Answer from the drawing. Dimensions are ordinates in mm from the lowest x, y and z of the part. A direction names the side the tool comes from. Round coordinates to 2 decimals unless told otherwise and drop trailing zeros. Loops run counter-clockwise (first coordinate to the right, second up) from the corner with the lowest first, then second, coordinate; pieces in that order, holes last.
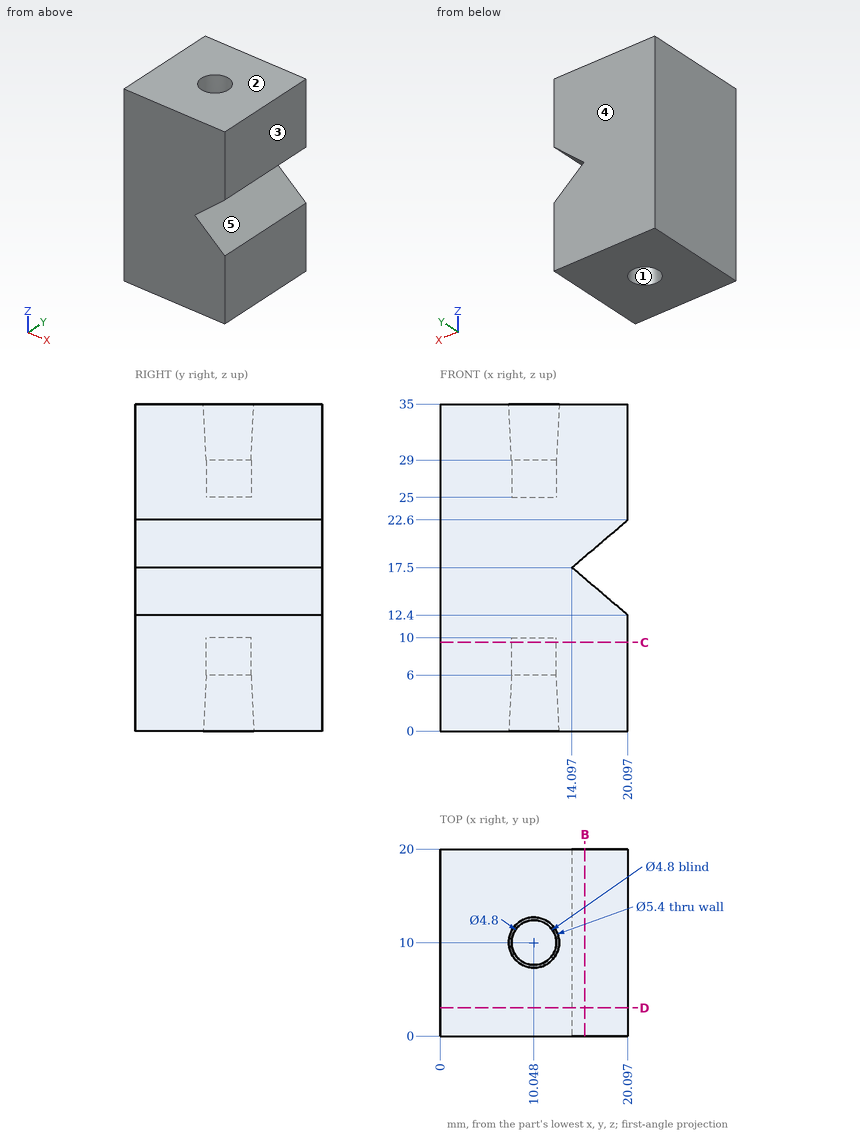
Item 1: For the marked faces 4 and 5, determine the directions among +Z, -Z, +X, -X, +Y, -Y from which every point of the face is accessible in a straight line to the end or side of a thin tool.
Item 2: Determine the mould class of the marked faces 1, 2 and 3 for opening direction X: pulls with the +X half, pulls with the -X half, needs draft (parallel to the pull), parting line crosses it, or undercut.
Item 3: Section B-B, the plane x = 15.5 is taken. Give the vertices of the cut face in (y, z).
Item 4: Section D-D, the plane y = 3 is taken. Give the vertices of the cut face in (x, z), plus the area to 3 significant figures.
Item 5: Straight lines are drawn through the part: line 1 (X direction, y = 11.25, z = 2.5) (1 decimal); line 2 (Y direction, x = 9.5, z = 8.5); line 3 (Z direction, x = 14.25, y = 4.75). For each, find the intervals that lie inside material, in ascending order.
Item 6: Each of these flat-tipped pins is pushed along its axis until it touches: P1, Ø3, axis at x = 10.05, y = 10, coming from the +Z side; P2, Ø2.5, axis at x = 10, y = 9, coming from the -Z side. Where does it stop, or does it pass through?
Item 7: Section C-C, the plane z = 9.5 is taken. Give the vertices of the cut face in (x, y).
Answer below:
1. face 4: +Z, -Z, +X, -X, +Y
1. face 5: +X, +Y, -Y
2. face 1: undercut
2. face 2: needs draft
2. face 3: pulls with the +X half
3. outline: (0, 0) - (20, 0) - (20, 16.31) - (0, 16.31) - close; (0, 18.69) - (20, 18.69) - (20, 35) - (0, 35) - close
4. outline: (0, 0) - (20.1, 0) - (20.1, 12.4) - (14.1, 17.5) - (20.1, 22.6) - (20.1, 35) - (0, 35) - close
4. area: 673 mm2
5. line 1: x = 0 to 7.8, 12.3 to 20.1
5. line 2: y = 0 to 7.66, 12.34 to 20
5. line 3: z = 0 to 17.37, 17.63 to 35
6. P1: stops at z = 25
6. P2: stops at z = 10
7. outline: (0, 0) - (20.1, 0) - (20.1, 20) - (0, 20) - close; hole circle Ø4.8 at (10.05, 10)
